Geometry check sheet. Reference: the model listing, model coordinates, mm. A direction names the side the tool comes from. Round coordinates to 2 decimals unless told otherwise and drop trailing zeros. Order: outer loops, then holes, each group sorted by start corner. A loop starts at its lowest first (then second) coordinate and runs counter-clockwise, first axis right, second up. Notation, with made-up numbers: (24, 27.25) - (35, 27.25) arc R38 cw to (35, 66.25) - close; hole circle Ø5 at (62, 71). An arc over 180 degrees is marked (long way). Use a Markdown table: item, result. Add a question column.
(1) Section check D-D on z = 11.5. Record the boundary of the cut face in (x, y).
(2) Access from +Z, -Z, +X, -X, +Y, -Y to the whole of each face (thin tool, end or side, straight path). Record for faces 5 (the face through (13, 0, 10.2)), 6 (the face through (0, -9.25, 3)), 7 (the face through (0, -8.05, 3)).
(3) Mould release check, pull along X, two halves, no side actions. Record for faces 1 (the face through (4, -9, 3)), 2 (the face through (-4, -9, 3)), 3 (the face through (0, 0, 1.2)), 4 (the face through (-3.7, 6.7, 3.2)): released by +X, released by -X, zero draft, split by the parting line, or undercut.
(4) Section check A-A on y = 8.5. Record the boundary of the cut face in (x, z).
(5) Section check B-B on x = -13. Record the boundary of the cut face in (y, z).
(6) Thickness scan on line 1 along Y through (x, z) = (21.25, 0.9); line 2 along Y through (x, z) = (-13, 11.7); line 3 along Z through (x, y) = (20.5, 4.25). Record the ranges inside material, lowest first. Write a range as [from, to].
(7) Gauge pin test, flat ends, axial feed: P1, Ø1.5, axis at x = 14.5, z = 4, coming from the -Y side; P2, Ø3, axis at x = 1, z = 3.5, coming from the +Y side; P3, Ø1.2, axis at x = -0.5, z = 4, coming from the -Y side. Record the tip position at first contact, or that the pin passes through.
(8) Section check C-C on z = 8.5. Record the boundary of the cut face in (x, y), then the cut area to 3 significant figures.
```python
from build123d import *

# Parameters (mm, degrees)
SKETCH_1_W          = 45.5
SKETCH_1_H          = 20.5
SKETCH_1_R          = 0.7
EXTRUDE_1_DEPTH     = 1.2
SKETCH_2_R          = 8
EXTRUDE_2_DEPTH     = 12
SKETCH_3_R          = 5
CUT_EXTRUDE_1_DEPTH = 3
FILLET_1_R          = 1
EXTRUDE_3_DEPTH     = 4
SKETCH_5_W          = 8
SKETCH_5_H          = 1.2
EXTRUDE_4_DEPTH     = 3


with BuildPart() as part:
    # 草图1 → 凸台-拉伸1 (new body)
    with BuildSketch(Plane.XY):
        Rectangle(SKETCH_1_W, SKETCH_1_H)
        with Locations((21.25, 8.5)):
            Circle(SKETCH_1_R, mode=Mode.SUBTRACT)
        with Locations((-21.25, 8.5)):
            Circle(SKETCH_1_R, mode=Mode.SUBTRACT)
        with Locations((-21.25, -8.5)):
            Circle(SKETCH_1_R, mode=Mode.SUBTRACT)
        with Locations((21.25, -8.5)):
            Circle(SKETCH_1_R, mode=Mode.SUBTRACT)
    extrude(amount=EXTRUDE_1_DEPTH)

    # 草图2 → 凸台-拉伸2 (add)
    with BuildSketch(Plane.XY.offset(1.2)):
        with Locations(Location((-13, 0, 0), (0, 0, 180))):
            Circle(SKETCH_2_R)
        with Locations(Location((13, 0, 0), (0, 0, 180))):
            Circle(SKETCH_2_R)
    extrude(amount=EXTRUDE_2_DEPTH)

    # 草图3 → 切除-拉伸1 (cut)
    with BuildSketch(Plane.XY.offset(13.2)):
        with Locations((-13, 0)):
            Circle(SKETCH_3_R)
        with Locations((13, 0)):
            Circle(SKETCH_3_R)
    extrude(amount=-CUT_EXTRUDE_1_DEPTH, mode=Mode.SUBTRACT)

    # 圆角1
    fillet_1_edges = [part.edges().sort_by_distance(p)[0] for p in [
        (-5, 0, 13.2),
        (21, 0, 13.2),
        (-18, 0, 13.2),
        (8, 0, 13.2),
    ]]
    fillet(fillet_1_edges, radius=FILLET_1_R)

    # 草图4 → 凸台-拉伸3 (add)
    with BuildSketch(Plane.XY.offset(1.2)):
        with BuildLine():
            Line((-2.5, 7.95), (2.5, 7.95))
            ThreePointArc((2.5, 7.95), (3.7, 6.75), (2.5, 5.55))
            Line((2.5, 5.55), (-2.5, 5.55))
            ThreePointArc((-2.5, 5.55), (-3.7, 6.75), (-2.5, 7.95))
        make_face()
    extrude(amount=EXTRUDE_3_DEPTH)

    # 草图5 → 凸台-拉伸4 (add)
    with BuildSketch(Plane.XY.offset(1.2)):
        with Locations((0, -8.65)):
            Rectangle(SKETCH_5_W, SKETCH_5_H)
    extrude(amount=EXTRUDE_4_DEPTH)


solid = part.part
```
Check sheet entries:
| question | item | result |
|---|---|---|
| 1 | outline | circle Ø16 at (-13, 0); circle Ø16 at (13, 0); hole circle Ø10 at (-13, 0); hole circle Ø10 at (13, 0) |
| 2 | face 5 | +Z |
| 2 | face 6 | +Z, +X, -X, -Y |
| 2 | face 7 | +Z, +X, -X |
| 3 | face 1 | released by +X |
| 3 | face 2 | released by -X |
| 3 | face 3 | undercut |
| 3 | face 4 | undercut |
| 4 | outline | (-22.75, 0) - (-21.95, 0) - (-21.95, 1.2) - (-22.75, 1.2) - close; (-20.55, 0) - (20.55, 0) - (20.55, 1.2) - (-20.55, 1.2) - close; (21.95, 0) - (22.75, 0) - (22.75, 1.2) - (21.95, 1.2) - close |
| 5 | outline | (-10.25, 0) - (10.25, 0) - (10.25, 1.2) - (8, 1.2) - (8, 12.2) arc R1 ccw to (7, 13.2) - (6, 13.2) arc R1 ccw to (5, 12.2) - (5, 10.2) - (-5, 10.2) - (-5, 12.2) arc R1 ccw to (-6, 13.2) - (-7, 13.2) arc R1 ccw to (-8, 12.2) - (-8, 1.2) - (-10.25, 1.2) - close |
| 6 | line 1 | y = [-10.25, -9.2], [-7.8, 7.8], [9.2, 10.25] |
| 6 | line 2 | y = [-8, -5], [5, 8] |
| 6 | line 3 | z = [0, 1.2] |
| 7 | P1 | stops at y = -7.96 |
| 7 | P2 | stops at y = 7.95 |
| 7 | P3 | stops at y = -9.25 |
| 8 | outline | circle Ø16 at (-13, 0); circle Ø16 at (13, 0) |
| 8 | area | 402 mm2 |
